```python
from build123d import *

# Parameters (mm, degrees)
BOSS_EXTRUDE1_DEPTH = 101.6
SKETCH2_R           = 3.175
CUT_EXTRUDE1_DEPTH  = 25.146
SKETCH3_R           = 3.175
CUT_EXTRUDE2_DEPTH  = 25.146


with BuildPart() as part:
    # Sketch1 → Boss-Extrude1 (new body)
    with BuildSketch(Plane.XY):
        Polygon((0, 44.45), (0, 0), (44.45, 0), (44.45, 6.35), (6.35, 6.35), (6.35, 44.45), align=None)
    extrude(amount=BOSS_EXTRUDE1_DEPTH)

    # Sketch2 → Cut-Extrude1 (cut)
    with BuildSketch(Plane(origin=(0, 6.35, 0), x_dir=(1, 0, 0), z_dir=(0, 1, 0))):
        with Locations(Location((35, -95.25, 0), (0, 0, 180))):
            Circle(SKETCH2_R)
        with Locations(Location((35, -6.35, 0), (0, 0, 180))):
            Circle(SKETCH2_R)
    extrude(amount=-CUT_EXTRUDE1_DEPTH, mode=Mode.SUBTRACT)

    # Sketch3 → Cut-Extrude2 (cut)
    with BuildSketch(Plane(origin=(6.35, 0, 0), x_dir=(0, 0, -1), z_dir=(1, 0, 0))):
        with Locations(Location((-12.7, 29.45, 0), (0, 0, 90))):
            Circle(SKETCH3_R)
        with Locations(Location((-63.5, 29.45, 0), (0, 0, 90))):
            Circle(SKETCH3_R)
        with Locations(Location((-88.9, 29.45, 0), (0, 0, 90))):
            Circle(SKETCH3_R)
        with Locations(Location((-38.1, 29.45, 0), (0, 0, 90))):
            Circle(SKETCH3_R)
    extrude(amount=-CUT_EXTRUDE2_DEPTH, mode=Mode.SUBTRACT)


solid = part.part
```
Model file for the job. Use its own axes, mm. A direction names the side the tool comes from. Round coordinates to 2 decimals unless told otherwise and drop trailing zeros. Write each loop counter-clockwise with the first axis right and the second up, starting at its lowest first coordinate (ties: lowest second). Pieces come first, ordered by that corner, then holes. Notation, with made-up numbers: M 76.5,19.5 L 125.5,19.5 A28 ccw 125.5,51.5 Z; hole C 14,-3.75 d7. An arc over 180 degrees is marked long. Put each result on its own line as item: value.
Item 1: Probe L1, parallel to Z at x = 1.5, y = 29.45 (3 decimals); L2, parallel to Z at x = 35, y = 3 (3 decimals); L3, parallel to X at y = 5, z = 95. List the from-to ranges inside material, lowest first. Write a range as from..to.
Responses:
L1: 0..9.525, 15.875..34.925, 41.275..60.325, 66.675..85.725, 92.075..101.6
L2: 0..3.175, 9.525..92.075, 98.425..101.6
L3: 0..31.83, 38.17..44.45
Item 2: Cut at A-A (x = 35). List the corners of the cut face in (y, z) (3 decimals), and give its area (3 significant figures).
Responses:
outline: M 0,0 L 6.35,0 L 6.35,3.175 L 0,3.175 Z; M 0,9.525 L 6.35,9.525 L 6.35,92.075 L 0,92.075 Z; M 0,98.425 L 6.35,98.425 L 6.35,101.6 L 0,101.6 Z
area: 565 mm²
Item 3: Cut at C-C (y = 30.5). List the corners of the cut face in (x, z).
Responses:
outline: M 0,0 L 6.35,0 L 6.35,9.7 L 0,9.7 Z; M 0,15.7 L 6.35,15.7 L 6.35,35.1 L 0,35.1 Z; M 0,41.1 L 6.35,41.1 L 6.35,60.5 L 0,60.5 Z; M 0,66.5 L 6.35,66.5 L 6.35,85.9 L 0,85.9 Z; M 0,91.9 L 6.35,91.9 L 6.35,101.6 L 0,101.6 Z
Item 4: Tool access for faces 4 (the flat face through (26, 6.35, 50)), 5 (the flat face through (22, 0, 50)): list every direction of +Z, -Z, +X, -X, +Y, -Y with a clear straight run to the whole face (end or side of a thin tool).
Responses:
face 4: +Z, -Z, +X, +Y
face 5: +Z, -Z, +X, -X, -Y
Item 5: Flat gauge pins, fed straight in: P1, Ø8, axis at x = 12, y = 38, coming from the +Z side; P2, Ø8.5, axis at y = 29.45, z = 88.9, coming from the +X side; P3, Ø2, axis at x = 32, z = 62, coming from the +Y side. Where does each tip first touch, or does it go through?
Responses:
P1: through
P2: x = 6.35
P3: y = 6.35
Item 6: Cut at B-B (z = 63.5). List the corners of the cut face in (x, y) (3 decimals), and give its area (3 significant figures).
Responses:
outline: M 0,0 L 44.45,0 L 44.45,6.35 L 6.35,6.35 L 6.35,26.275 L 0,26.275 Z; M 0,32.625 L 6.35,32.625 L 6.35,44.45 L 0,44.45 Z
area: 484 mm²
Item 7: Mould opens along Y. For faces 1 (the cylindrical face through (3.219, 27.11, 65.646)), 2 (the flat face through (3, 44.45, 50)), 3 (the flat face through (44.45, 3, 50)) say: +Y half, -Y half, draft (parallel to the pull), parting line (faces both ways), or undercut.
Responses:
face 1: undercut
face 2: +Y half
face 3: draft
Item 8: Cut at D-D (z = 81.5). List the corners of the cut face in (x, y), and give its area (3 significant figures).
Responses:
outline: M 0,0 L 44.45,0 L 44.45,6.35 L 6.35,6.35 L 6.35,44.45 L 0,44.45 Z
area: 524 mm²
